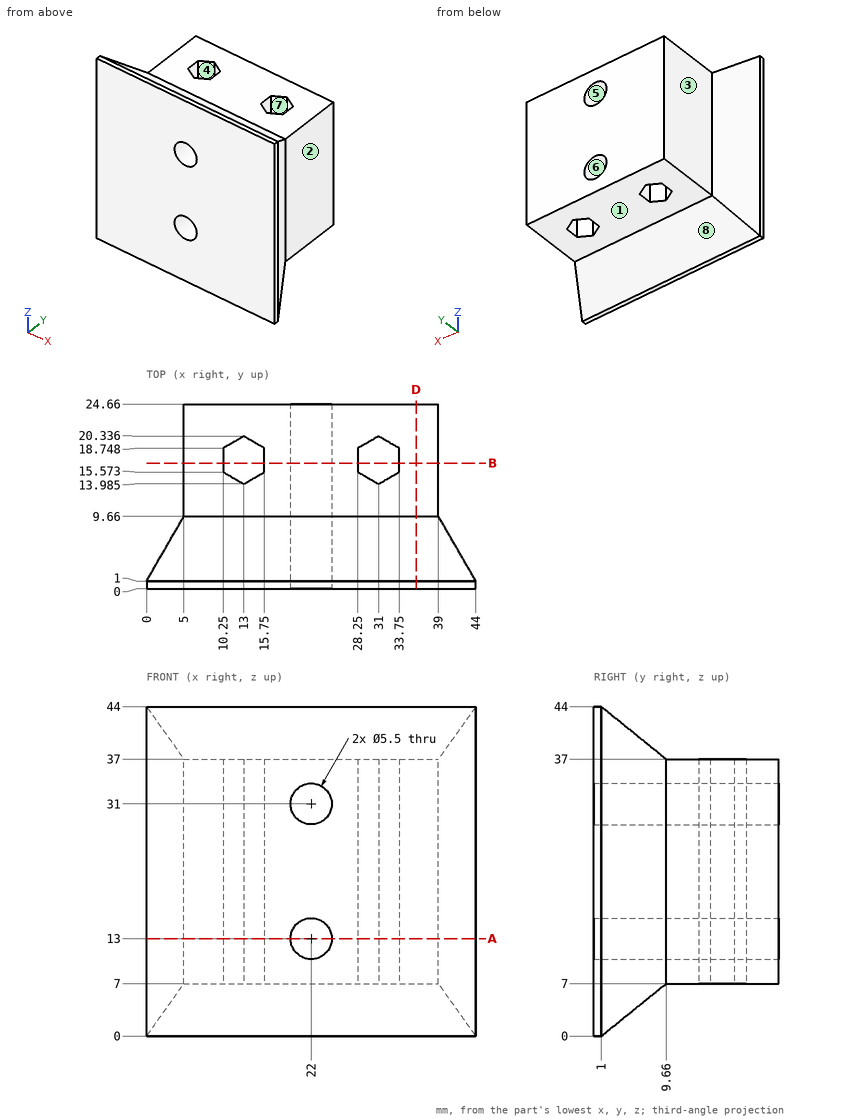
Input: dimensioned drawing with shaded views. Units: mm. Origin: part minimum x, y, z. A direction names the side the tool comes from. Give positions to 0.01 mm unless a question says otherwise; leave off trailing zeros. Write each loop counter-clockwise with the first axis right and the second up, starting at its lowest first coordinate (ties: lowest second). Pieces come first, ordered by that corner, then holes. Notation, with made-up numbers: M 1,62 L 51,62 A24 ccw 51,93 Z; hole C -39,70.5 d8. An arc over 180 degrees is marked long. Return JSON: item names as keys, results as strings. Group by question number.
1) Pull-direction query (Z, two-part tool) for the marked faces 5, 6, 7 and 8; classes: pulls with the +Z half, pulls with the -Z half, needs draft (parallel to the pull), parting line crosses it, or undercut.
2) Pin query (flat end, axial travel): P1, Ø12, axis at y = 16, z = 21.5, coming from the +X side; P2, Ø1, axis at x = 24.5, y = 7, coming from the -Z side (1 decimal); P3, Ø7.5, axis at y = 15.5, z = 29, coming from the -X side; P4, Ø3.5, axis at x = 22, z = 13, coming from the +Y side. Return the tip coordinate at first contact, or that it passes through.
3) Cut plane D-D, the plane x = 36. Output: boundary loops of the cut face in (y, z).
4) Cut plane A-A, the plane z = 13. Give the number of separate pieces and of enclosed holes in the cut face, plus the area to 3 significant figures.
5) Material intervals for line 1 along Z through (x, y) = (22, 16); line 2 along Y through (x, z) = (31, 22) (1 decimal); line 3 along X through (y, z) = (10.25, 13), sorted ascending. Write a range as [from, to].
6) Cut plane B-B, the plane y = 16.75. Output: boundary loops of the cut face in (x, z).
7) Set-up query: the marked faces 1, 2, 3 and 4. Return all of +Z, -Z, +X, -X, +Y, -Y with unobstructed straight access to the full face (end or side cutting, diameter ignored); none if empty.
Recorded:
{
 "1": {"face 5": "undercut", "face 6": "undercut", "face 7": "needs draft", "face 8": "pulls with the -Z half"},
 "2": {"P1": "stops at x = 39", "P2": "stops at z = 4.4", "P3": "stops at x = 5", "P4": "passes through"},
 "3": {"outline": "M 0,0 L 1,0 L 9.66,7 L 24.66,7 L 24.66,37 L 9.66,37 L 1,44 L 0,44 Z"},
 "4": {"separate pieces": "2", "enclosed holes": "2", "area": "704 mm²"},
 "5": {"line 1": "z = [7, 10.25], [15.75, 28.25], [33.75, 37]", "line 2": "y = [0, 14], [20.3, 24.7]", "line 3": "x = [5, 19.25], [24.75, 39]"},
 "6": {"outline": "M 5,7 L 10.25,7 L 10.25,37 L 5,37 Z; M 15.75,7 L 28.25,7 L 28.25,37 L 15.75,37 Z; M 33.75,7 L 39,7 L 39,37 L 33.75,37 Z; hole C 22,13 d5.5; hole C 22,31 d5.5"},
 "7": {"face 1": "-Z, +X, -X, +Y", "face 2": "+Z, -Z, +X, +Y", "face 3": "+Z, -Z, -X, +Y", "face 4": "+Z, -Z"}
}
